Study the drawing (mm; zero at the part's minimum x, y, z) and answer. Coordinates: 2 decimals unless noted, no trailing zeros. Write each loop counter-clockwise with the first axis right and the second up, starting at its lowest first coordinate (ties: lowest second). Pieces come first, ordered by that corner, then holes. Notation, with made-up numbers: (84.5, 42) - (105.5, 42) arc R6 cw to (105.5, 52) - close; hole circle Ø7 at (-22, -30). An arc over 180 degrees is marked (long way). One line per item, written item: value.
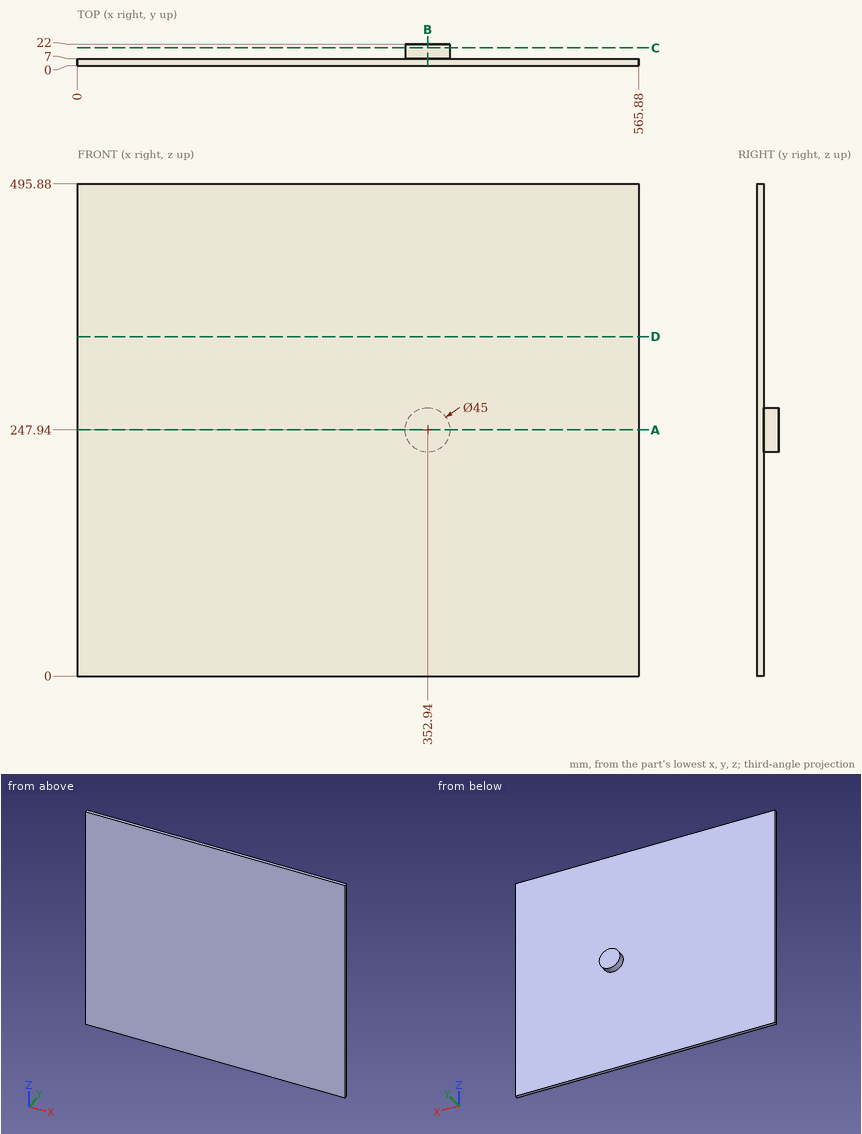
Item 1: Section D-D, the plane z = 342 is taken. Determine the outline of the cut face in (x, y).
Evaluation:
outline: (0, 0) - (565.88, 0) - (565.88, 7) - (0, 7) - close
Item 2: Consider probe 1 along Y at (x, z) = (210.5, 80.5); probe 2 along Z at (x, y) = (354.5, 7.75); probe 3 along Z at (x, y) = (352.5, 10). Determine where each line is inside the solid, lowest interval first.
Evaluation:
probe 1: y = 0 to 7
probe 2: z = 225.49 to 270.39
probe 3: z = 225.44 to 270.44
Item 3: Section C-C, the plane y = 18 is taken. Determine the outline of the cut face in (x, z).
Evaluation:
outline: circle Ø45 at (352.94, 247.94)
Item 4: Section B-B, the plane x = 352.94 is taken. Determine the outline of the cut face in (y, z).
Evaluation:
outline: (0, 0) - (7, 0) - (7, 225.44) - (22, 225.44) - (22, 270.44) - (7, 270.44) - (7, 495.88) - (0, 495.88) - close
Item 5: Section A-A, the plane z = 247.94 is taken. Determine the outline of the cut face in (x, y).
Evaluation:
outline: (0, 0) - (565.88, 0) - (565.88, 7) - (375.44, 7) - (375.44, 22) - (330.44, 22) - (330.44, 7) - (0, 7) - close
Item 6: Given pin 1 (10 mm diameter, centred on x = 335.5, y = 13.5, fed in from -Z); pin 2 (6 mm diameter, centred on x = 387, y = 11.5, fed in from +Z); pin 3 (10 mm diameter, centred on x = 284, z = 87.5, fed in from +Y), each flat-ended and moving along its own axis, determine where each tip first touches the part or whether it passes through.
Evaluation:
pin 1: stops at z = 229.19
pin 2: passes through
pin 3: stops at y = 7
